Source: CAD feature listing. Evaluate the final solid. Frame: model axes, mm. Coordinates: 2 decimals unless noted, no trailing zeros. Loops run counter-clockwise (first coordinate to the right, second up) from the corner with the lowest first, then second, coordinate; pieces in that order, holes last. Notation, with made-up numbers: (69, -40) -> (89, -40) arc R18 ccw to (89, -19) -> close; hole circle Ø6 at (63, -26.5). An arc over 180 degrees is marked (long way). Answer as a JSON object with one key per item and string values. Group by question number.
from build123d import *

# Parameters (mm, degrees)
F0_R     = 6.35
F0_R_2   = 12.7
F1_DEPTH = 19.05


with BuildPart() as f1:
    # F0 (on Front) → F1 (new body)
    with BuildSketch(Plane.XZ):
        with BuildLine():
            ThreePointArc((50.8, 12.7), (23.379701, 23.379701), (12.7, 50.8))
            ThreePointArc((12.7, 50.8), (0, 63.5), (-12.7, 50.8))
            ThreePointArc((-12.7, 50.8), (-23.379701, 23.379701), (-50.8, 12.7))
            ThreePointArc((-50.8, 12.7), (-63.5, 0), (-50.8, -12.7))
            ThreePointArc((-50.8, -12.7), (-23.379701, -23.379701), (-12.7, -50.8))
            ThreePointArc((-12.7, -50.8), (0, -63.5), (12.7, -50.8))
            ThreePointArc((12.7, -50.8), (23.379701, -23.379701), (50.8, -12.7))
            ThreePointArc((50.8, -12.7), (63.5, 0), (50.8, 12.7))
        make_face()
        with Locations((0, -50.8)):
            Circle(F0_R, mode=Mode.SUBTRACT)
        with Locations((-50.8, 0)):
            Circle(F0_R, mode=Mode.SUBTRACT)
        Circle(F0_R_2, mode=Mode.SUBTRACT)
        with Locations((50.8, 0)):
            Circle(F0_R, mode=Mode.SUBTRACT)
        with Locations((0, 50.8)):
            Circle(F0_R, mode=Mode.SUBTRACT)
    extrude(amount=F1_DEPTH)


solid = f1.part
1. Section query C-C on y = -7.5. Return loops of the section in (x, z).
2. Mould query, pull axis X, two halves, no side actions, for faces 1 (the face through (9.1, 0, -9.1)), 2 (the face through (-0.8, -9.4, -44.5)), 3 (the face through (63.497, -9.392, -0.279)), 4 (the face through (0.279, -9.392, 63.497)). Classes: pulls with the +X half, pulls with the -X half, needs draft (parallel to the pull), parting line crosses it, or undercut.
3. Pin query (flat end, axial travel): pin 1 Ø1.5 at (y, z) = (-9.5, 38) entering from -X; pin 2 Ø10 at (x, y) = (0.5, -3.5) entering from +Z; pin 3 Ø5 at (x, y) = (-50, -13) entering from -Z; pin 4 Ø7.5 at (x, z) = (0, -50.8) entering from -Y. Return the tip coordinate at first contact, or that it passes through.
4. Section query A-A on z = 0. Return loops of the section in (x, y), then the cut area to 3 significant figures.
5. Section query B-B on x = 0. Return loops of the section in (y, z), then the cut area to 3 significant figures.
6. Ray query, L1, parallel to Z at x = 0, y = -11.5; L2, parallel to X at y = -16.5, z = 3; L3, parallel to Z at x = 5, y = -17.75. Return the intervals inside material, ascending.
7. Section query D-D on x = 53. Return loops of the section in (y, z).
Solved:
{
 "1": {"outline": "(-50.8, -12.7) arc R36.58 cw to (-12.7, -50.8) arc R12.7 ccw to (12.7, -50.8) arc R36.58 cw to (50.8, -12.7) arc R12.7 ccw to (50.8, 12.7) arc R36.58 cw to (12.7, 50.8) arc R12.7 ccw to (-12.7, 50.8) arc R36.58 cw to (-50.8, 12.7) arc R12.7 ccw to start; hole circle Ø12.7 at (-50.8, 0); hole circle Ø25.4 at (0, 0); hole circle Ø12.7 at (0, -50.8); hole circle Ø12.7 at (0, 50.8); hole circle Ø12.7 at (50.8, 0)"},
 "2": {"face 1": "needs draft", "face 2": "undercut", "face 3": "pulls with the +X half", "face 4": "parting line crosses it"},
 "3": {"pin 1": "x = -14.69", "pin 2": "z = 63.5", "pin 3": "z = -12.71", "pin 4": "through"},
 "4": {"outline": "(-63.5, -19.05) -> (-57.15, -19.05) -> (-57.15, 0) -> (-63.5, 0) -> close; (-44.45, -19.05) -> (-12.7, -19.05) -> (-12.7, 0) -> (-44.45, 0) -> close; (12.7, -19.05) -> (44.45, -19.05) -> (44.45, 0) -> (12.7, 0) -> close; (57.15, -19.05) -> (63.5, -19.05) -> (63.5, 0) -> (57.15, 0) -> close", "area": "1,450 mm^2"},
 "5": {"outline": "(-19.05, -63.5) -> (0, -63.5) -> (0, -57.15) -> (-19.05, -57.15) -> close; (-19.05, -44.45) -> (0, -44.45) -> (0, -12.7) -> (-19.05, -12.7) -> close; (-19.05, 12.7) -> (0, 12.7) -> (0, 44.45) -> (-19.05, 44.45) -> close; (-19.05, 57.15) -> (0, 57.15) -> (0, 63.5) -> (-19.05, 63.5) -> close", "area": "1,450 mm^2"},
 "6": {"L1": "-63.5 to -57.15, -44.45 to -12.7, 12.7 to 44.45, 57.15 to 63.5", "L2": "-63.14 to -56.4, -45.2 to -12.34, 12.34 to 45.2, 56.4 to 63.14", "L3": "-62.47 to -54.71, -46.89 to -11.67, 11.67 to 46.89, 54.71 to 62.47"},
 "7": {"outline": "(-19.05, -12.51) -> (0, -12.51) -> (0, -5.96) -> (-19.05, -5.96) -> close; (-19.05, 5.96) -> (0, 5.96) -> (0, 12.51) -> (-19.05, 12.51) -> close"}
}
